Could you check a few things on this model? Use its own coordinates, in mm. A direction names the side the tool comes from. Give positions to 0.01 mm unless a question says otherwise; leave off trailing zeros. Use a Markdown table: item, result. Add a question column.
1) Suppose I cut it at A-A on y = 9. Count the separate pieces of the cut face and the enclosed holes in it, and give its area (4 significant figures).
2) Which directions (+Z, -Z, +X, -X, +Y, -Y) give clear straight access to the entire face, cutting with the end or side of a thin tool? Please do faces 5 (the flat face through (12, -25.4, 7)), 6 (the flat face through (-5.2, 10, 7)), 7 (the flat face through (-10.1, -16, 7)).
3) Will this pin go through, and if not, where does the flat tip stop? pin 1 Ø0.6 at (x, z) = (28.5, 7) entering from +Y.
4) If I drill on line 1 along Y through (x, z) = (10.5, 2), over which ranges is the centre line in solid material (lowest first)? Write a range as [from, to].
5) We'd pull the mould along X, two halves only. Please class faces 1 (the flat face through (-4.2, -16, 7)), 2 (the flat face through (-20.7, 10, 7)), 3 (the flat face through (1.5, -25.4, 7.4)), 4 (the flat face through (31.3, 0, 7)): +X half, -X half, draft (parallel to the pull), parting line (faces both ways), or undercut.
```python
from build123d import *

# Parameters (mm, degrees)
F1_DEPTH = 15


with BuildPart() as f1:
    # F0 (on Top) → F1 (new body)
    with BuildSketch(Plane.XY):
        Polygon((-23.1, 25.4), (-23.4, 25.4), (-23.4, -25.4), (-23.1, -25.4), (-23.1, -5.4), (-21.1, -5.4), (-21.1, -25.4), (-20.7, -25.4), (-20.7, -5.4), (-18.7, -5.4), (-18.7, -25.4), (-18.2, -25.4), (-18.2, -5.4), (-16.2, -5.4), (-16.2, -25.4), (-15.6, -25.4), (-15.6, -5.4), (-13.6, -5.4), (-13.6, -25.4), (-12.9, -25.4), (-12.9, -5.4), (-10.9, -5.4), (-10.9, -25.4), (-10.1, -25.4), (-10.1, -5.4), (-8.1, -5.4), (-8.1, -25.4), (-7.2, -25.4), (-7.2, -5.4), (-5.2, -5.4), (-5.2, -25.4), (-4.2, -25.4), (-4.2, -5.4), (-2.2, -5.4), (-2.2, -25.4), (-1.1, -25.4), (-1.1, -5.4), (0.9, -5.4), (0.9, -25.4), (2.1, -25.4), (2.1, -5.4), (4.1, -5.4), (4.1, -25.4), (5.4, -25.4), (5.4, -5.4), (7.4, -5.4), (7.4, -25.4), (8.8, -25.4), (8.8, -5.4), (10.8, -5.4), (10.8, -25.4), (12.3, -25.4), (12.3, -5.4), (14.3, -5.4), (14.3, -25.4), (15.9, -25.4), (15.9, -5.4), (17.9, -5.4), (17.9, -25.4), (19.6, -25.4), (19.6, -5.4), (21.6, -5.4), (21.6, -25.4), (23.4, -25.4), (23.4, -5.4), (25.4, -5.4), (25.4, -25.4), (27.3, -25.4), (27.3, -5.4), (29.3, -5.4), (29.3, -25.4), (31.3, -25.4), (31.3, -5.4), (31.3, -5.2), (31.3, 25.4), (29.3, 25.4), (29.3, -5.2), (27.3, -5.2), (27.3, 25.4), (25.4, 25.4), (25.4, -5.2), (23.4, -5.2), (23.4, 25.4), (21.6, 25.4), (21.6, -5.2), (19.6, -5.2), (19.6, 25.4), (17.9, 25.4), (17.9, -5.2), (15.9, -5.2), (15.9, 25.4), (14.3, 25.4), (14.3, -5.2), (12.3, -5.2), (12.3, 25.4), (10.8, 25.4), (10.8, -5.2), (8.8, -5.2), (8.8, 25.4), (7.4, 25.4), (7.4, -5.2), (5.4, -5.2), (5.4, 25.4), (4.1, 25.4), (4.1, -5.2), (2.1, -5.2), (2.1, 25.4), (0.9, 25.4), (0.9, -5.2), (-1.1, -5.2), (-1.1, 25.4), (-2.2, 25.4), (-2.2, -5.2), (-4.2, -5.2), (-4.2, 25.4), (-5.2, 25.4), (-5.2, -5.2), (-7.2, -5.2), (-7.2, 25.4), (-8.1, 25.4), (-8.1, -5.2), (-10.1, -5.2), (-10.1, 25.4), (-10.9, 25.4), (-10.9, -5.2), (-12.9, -5.2), (-12.9, 25.4), (-13.6, 25.4), (-13.6, -5.2), (-15.6, -5.2), (-15.6, 25.4), (-16.2, 25.4), (-16.2, -5.2), (-18.2, -5.2), (-18.2, 25.4), (-18.7, 25.4), (-18.7, -5.2), (-20.7, -5.2), (-20.7, 25.4), (-21.1, 25.4), (-21.1, -5.2), (-23.1, -5.2), align=None)
    extrude(amount=F1_DEPTH)


solid = f1.part
```
Answer block:
| question | item | result |
|---|---|---|
| 1 | separate pieces | 18 |
| 1 | enclosed holes | 0 |
| 1 | area | 310.5 mm^2 |
| 2 | face 5 | +Z, -Z, +X, -X, -Y |
| 2 | face 6 | +Z, -Z, +Y |
| 2 | face 7 | +Z, -Z, -Y |
| 3 | pin 1 | stops at y = -5.2 |
| 4 | line 1 | y = [-5.4, -5.2] |
| 5 | face 1 | undercut |
| 5 | face 2 | undercut |
| 5 | face 3 | draft |
| 5 | face 4 | +X half |
